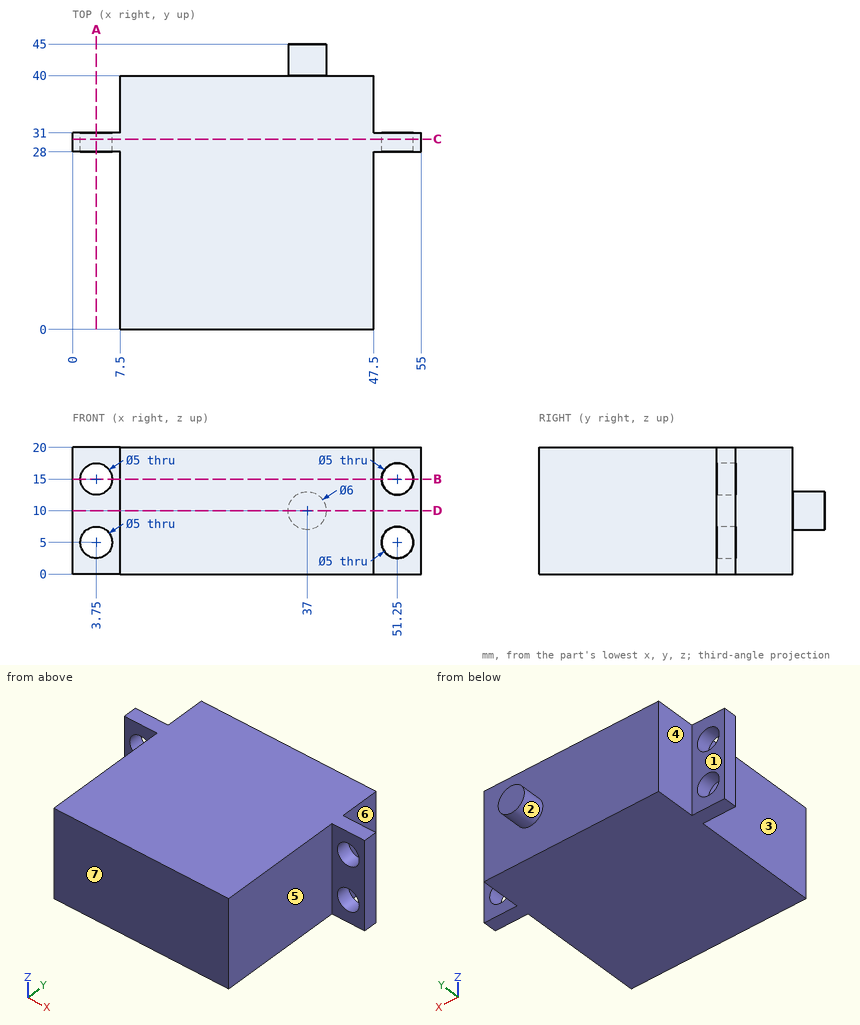
Check sheet for the drawn part. Datum: minimum x, y, z corner. Units: mm. A direction names the side the tool comes from. Round coordinates to 2 decimals unless told otherwise and drop trailing zeros. Write each loop counter-clockwise with the first axis right and the second up, starting at its lowest first coordinate (ties: lowest second). Pieces come first, ordered by that corner, then holes. Notation, with made-up numbers: (75.5, 28.5) -> (123.5, 28.5) arc R35 cw to (123.5, 65.5) -> close; hole circle Ø10 at (77.5, -20). An arc over 180 degrees is marked (long way). Write each question's results on one line, items separated by ' | '.
Q1. Sectioned sample at D-D, the plane z = 10. Record the boundary of the cut face in (x, y), and give its area (4 significant figures).
Derived:
outline: (0, 28) -> (7.5, 28) -> (7.5, 0) -> (47.5, 0) -> (47.5, 28) -> (55, 28) -> (55, 31) -> (47.5, 31) -> (47.5, 40) -> (40, 40) -> (40, 45) -> (34, 45) -> (34, 40) -> (7.5, 40) -> (7.5, 31) -> (0, 31) -> close | area: 1,675 mm²
Q2. Sectioned sample at A-A, the plane x = 3.75. Record the boundary of the cut face in (y, z), and give its area (3 significant figures).
Derived:
outline: (28, 0) -> (31, 0) -> (31, 2.5) -> (28, 2.5) -> close; (28, 7.5) -> (31, 7.5) -> (31, 12.5) -> (28, 12.5) -> close; (28, 17.5) -> (31, 17.5) -> (31, 20) -> (28, 20) -> close | area: 30.0 mm²
Q3. Sectioned sample at C-C, the plane y = 30. Record the boundary of the cut face in (x, z), and give its area (3 significant figures).
Derived:
outline: (0, 0) -> (55, 0) -> (55, 20) -> (0, 20) -> close; hole circle Ø5 at (3.75, 5); hole circle Ø5 at (3.75, 15); hole circle Ø5 at (51.25, 5); hole circle Ø5 at (51.25, 15) | area: 1,020 mm²
Q4. Draft check along X on the marked faces 1, 2 and 3. Enter one of: released by +X, released by -X, zero draft, split by the parting line, or undercut.
Derived:
face 1: zero draft | face 2: split by the parting line | face 3: released by -X
Q5. Sectioned sample at B-B, the plane z = 15. Record the boundary of the cut face in (x, y).
Derived:
outline: (0, 28) -> (1.25, 28) -> (1.25, 31) -> (0, 31) -> close; (6.25, 28) -> (7.5, 28) -> (7.5, 0) -> (47.5, 0) -> (47.5, 28) -> (48.75, 28) -> (48.75, 31) -> (47.5, 31) -> (47.5, 40) -> (7.5, 40) -> (7.5, 31) -> (6.25, 31) -> close; (53.75, 28) -> (55, 28) -> (55, 31) -> (53.75, 31) -> close
Q6. Access from +Z, -Z, +X, -X, +Y, -Y to the whole of each face (thin tool, end or side, straight path). Record for the marked faces 4, 5, 6 and 7.
Derived:
face 4: +Z, -Z, -X, +Y | face 5: +Z, -Z, +X, -Y | face 6: +Z, -Z, +X, +Y | face 7: +Z, -Z, +X, -X, -Y
Q7. Go/stop test with flat-tipped pins: pin 1 Ø4.5 at (y, z) = (33.5, 10.5) entering from +X; pin 2 Ø2 at (x, z) = (51, 5.5) entering from -Y; pin 3 Ø4 at (x, z) = (2.5, 14.5) entering from +Y; pin 4 Ø6 at (x, z) = (51.25, 5) entering from -Y. Record where each tip stops, or that it passes through.
Derived:
pin 1: stops at x = 47.5 | pin 2: passes through | pin 3: stops at y = 31 | pin 4: stops at y = 28
Q8. Thickness scan on probe 1 along X at (y, z) = (28.9, 15); probe 2 along Z at (x, y) = (51.25, 29.45); probe 3 along Y at (x, z) = (33, 12.75). Record the ranges inside material, lowest first.
Derived:
probe 1: x = 0 to 1.25, 6.25 to 48.75, 53.75 to 55 | probe 2: z = 0 to 2.5, 7.5 to 12.5, 17.5 to 20 | probe 3: y = 0 to 40
